Verification items for this drawing (mm, ordinates from the low corner). A direction names the side the tool comes from. Round coordinates to 2 decimals unless told otherwise and drop trailing zeros. Order: outer loops, then holes, each group sorted by start corner. A loop starts at its lowest first (then second) coordinate and runs counter-clockwise, first axis right, second up. Notation, with made-up numbers: M -23,19 L 0,19 A15 ccw 0,39 Z; hole C 13,8 d2. An arc over 180 degrees is marked long. One line per item, written item: value. Start each with the question number.
(1) Thickness scan on L1, parallel to Z at x = 4, y = 6.25; L2, parallel to X at y = 3.5, z = 3.25; L3, parallel to Y at x = 3.4, z = 6.25. Record the ranges inside material, lowest first.
(2) Cross-section at A-A, the plane y = 4.25. Enter the section's corners in (x, z), and give its area (3 significant figures).
(3) Cross-section at C-C, the plane z = 1. Enter the section's corners in (x, y), and give its area (3 significant figures).
(4) Access from +Z, -Z, +X, -X, +Y, -Y to the whole of each face (thin tool, end or side, straight path). Record for the marked faces 1 and 2.
(5) Cross-section at B-B, the plane x = 3.35. Enter the section's corners in (y, z), and give its area (3 significant figures).
(6) Cross-section at D-D, the plane y = 0.75. Enter the section's corners in (x, z).
(7) Depth check by flat-ended pin: pin 1 Ø1 at (y, z) = (3, 2) entering from -X; pin 2 Ø4 at (y, z) = (2.5, 5.5) entering from -X. Enter the tip coordinate at first touch or a pass-through.
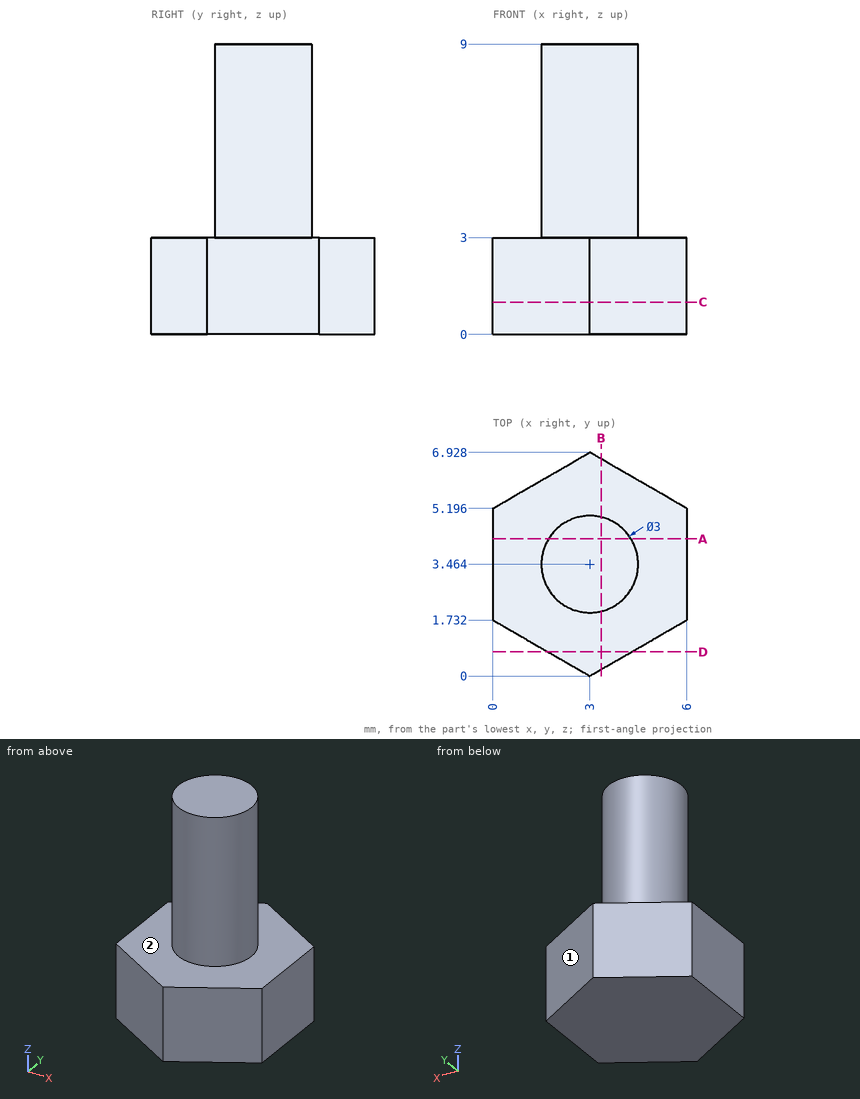
Values found:
1. L1: 0 to 3
1. L2: 1.5 to 4.5
1. L3: 2.02 to 4.91
2. outline: M 0,0 L 6,0 L 6,3 L 4.28,3 L 4.28,9 L 1.72,9 L 1.72,3 L 0,3 Z
2. area: 33.3 mm^2
3. outline: M 0,1.73 L 3,0 L 6,1.73 L 6,5.2 L 3,6.93 L 0,5.2 Z
3. area: 31.2 mm^2
4. face 1: +Z, -Z, +X, +Y
4. face 2: +Z
5. outline: M 0.2,0 L 6.73,0 L 6.73,3 L 4.92,3 L 4.92,9 L 2.01,9 L 2.01,3 L 0.2,3 Z
5. area: 37.1 mm^2
6. outline: M 1.7,0 L 4.3,0 L 4.3,3 L 1.7,3 Z
7. pin 1: x = 0
7. pin 2: x = 1.5
